Design review of the part built by this model. Coordinates are the model's own, in mm. A direction names the side the tool comes from. Coordinates: 2 decimals unless noted, no trailing zeros. Loops run counter-clockwise (first coordinate to the right, second up) from the corner with the lowest first, then second, coordinate; pieces in that order, holes last.
Q1. Add section D-D on x = 25.5. Give the boundary of the cut face in (y, z), and give its area (3 significant figures).
Q2. Add section A-A on z = 6. Give the boundary of the cut face in (x, y), and give its area (3 significant figures).
Q3. Wall thickness on probe 1 along X at (y, z) = (80.5, 40.5); probe 2 along Y at (x, z) = (25, 16.5); probe 3 along Y at (x, z) = (108, 42): over which ranges is each line inside the solid? List them lowest first.
Q4. Machinability: for faces 1 (the face through (30, -32, 22)), 2 (the face through (26, 184.15, 22)), 3 (the face through (50.8, 123, 22)), which of the approach directions +Z, -Z, +X, -X, +Y, -Y give a long, thin tool a straight path to every point of the face, cutting with its end or side? Answer none if there is none.
Q5. For P1, Ø22, axis at x = 88, z = 12.5, coming from the +Y side; P2, Ø3, axis at x = 63, z = 10.5, coming from the -Y side; P3, Ø3, axis at y = 86, z = 33.5, coming from the +X side, all flat-tipped, find the tip position at first contact; note any pin that passes through.
Q6. Add section B-B on x = 110.5. Give the boundary of the cut face in (y, z).
Q7. Add section C-C on y = 111. Give the boundary of the cut face in (x, z).
Autodesk Inventor part; units mm, degrees
ref_plane "YZ Plane" through (0, 0, 0) normal (1, 0, 0) x (0, 1, 0)
ref_plane "XZ Plane" through (0, 0, 0) normal (0, 1, 0) x (-1, 0, 0)
ref_plane "XY Plane" through (0, 0, 0) normal (0, 0, 1) x (1, 0, 0)
sketch "Sketch1" plane through (0, 0, 0) normal (0, 0, 1) x (1, 0, 0)
  line L0 (0, 0) -> (50.8, 0)
  line L1 (50.8, 63) -> (50.8, 184.15)
  line L2 (50.8, 184.15) -> (0, 184.15)
  line L3 (0, 184.15) -> (0, 0)
  line L4 (50.8, 0) -> (120.8, 0)
  line L5 (120.8, 0) -> (120.8, 63)
  line L6 (120.8, 63) -> (50.8, 63)
  line L7 (50.8, 63) -> (50.8, 0)
  dimension "d0" = 50.8
  dimension "d2" = 70
  dimension "d3" = 63
extrude "Extrusion2" add sketch "Sketch1" along normal blind 44.1
sketch "Sketch3" plane through (0, 0, 0) normal (0, -1, 0) x (1, 0, 0)
  line L0 (120.8, 44.1) -> (0, 44.1)
  line L1 (0, 0) -> (0, 44.1)
  line L2 (0, 0) -> (120.8, 0)
  line L3 (120.8, 0) -> (120.8, 44.1)
sketch "Sketch4" plane through (0, 0, 0) normal (0, -1, 0) x (1, 0, 0)
  circle A0 centre (21.61, 22.21) radius 12.5
  dimension "d8" = 25
extrude "Extrusion3" add sketch "Sketch4" along normal blind 32
sketch "Sketch5" plane through (21.61, -32, 22.21) normal (0, -1, 0) x (1, 0, 0)
  circle A0 centre (0, 0) radius 12.5
  circle A1 centre (0, 0) radius 8
  point P0 (-21.61, -22.21)
  dimension "d12" = 16
extrude "Extrusion4" add sketch "Sketch5" along normal blind 17.64 contours A1
sketch "Sketch6" plane through (21.61, -49.64, 22.21) normal (0, -1, 0) x (1, 0, 0)
  circle A0 centre (0, 0) radius 8
  circle A1 centre (0, 0) radius 1.5
  point P0 (-21.61, -22.21)
  dimension "d15" = 3
extrude "Extrusion5" add sketch "Sketch6" along normal blind 7 contours A1
sketch "Sketch7" plane through (21.61, -56.64, 22.21) normal (0, -1, 0) x (1, 0, 0)
  circle A0 centre (0, 0) radius 1.5
  point P0 (-21.61, -22.21)
properties part number "tool Part1"
Entries:
1. outline: (-49.64, 15.22) - (-32, 15.22) - (-32, 10.33) - (0, 10.33) - (0, 0) - (184.15, 0) - (184.15, 44.1) - (0, 44.1) - (0, 34.09) - (-32, 34.09) - (-32, 29.2) - (-49.64, 29.2) - close
1. area: 9,130 mm2
2. outline: (0, 0) - (120.8, 0) - (120.8, 63) - (50.8, 63) - (50.8, 184.15) - (0, 184.15) - close
2. area: 13,800 mm2
3. probe 1: x = 0 to 50.8
3. probe 2: y = -49.64 to 184.15
3. probe 3: y = 0 to 63
4. face 1: -Y
4. face 2: +Z, -Z, +X, -X, +Y
4. face 3: +Z, -Z, +X, +Y
5. P1: stops at y = 63
5. P2: stops at y = 0
5. P3: stops at x = 50.8
6. outline: (0, 0) - (63, 0) - (63, 44.1) - (0, 44.1) - close
7. outline: (0, 0) - (50.8, 0) - (50.8, 44.1) - (0, 44.1) - close
